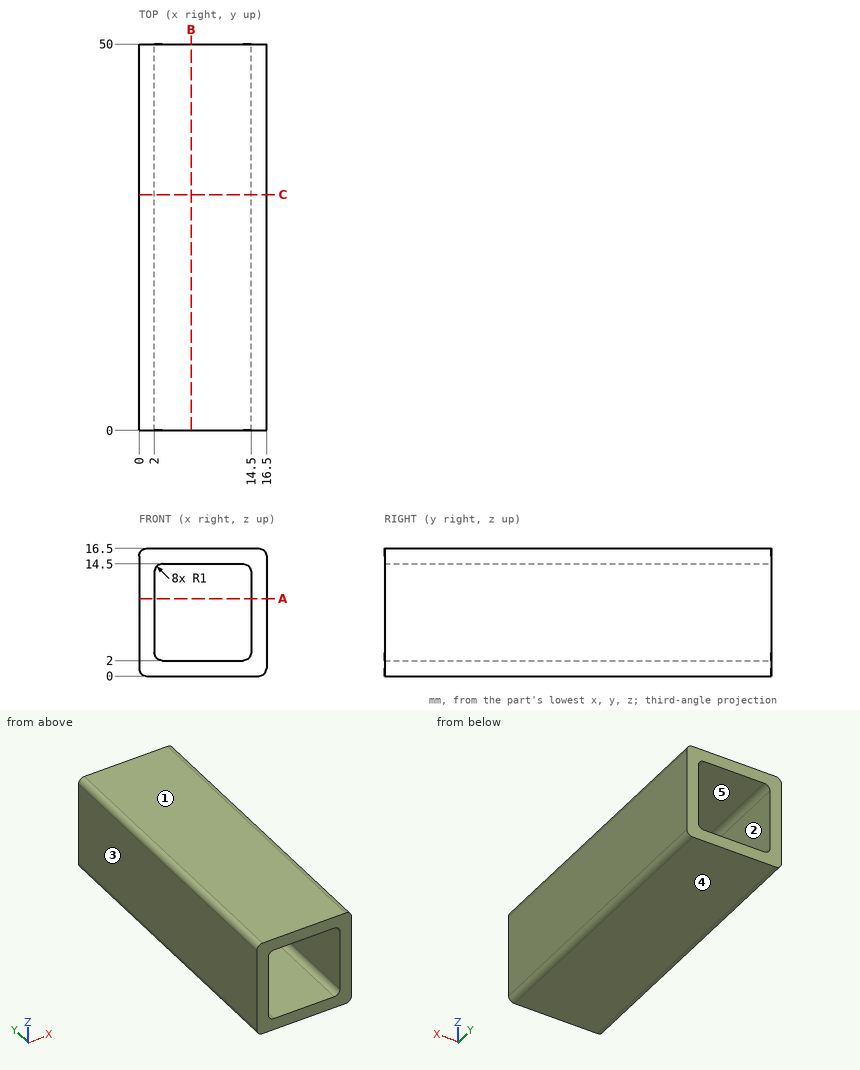
Could you check a few things on this drawing? It's one solid part, dimensions in mm from its lowest x, y, z. A direction names the side the tool comes from. Give positions to 0.01 mm unless a question says otherwise; leave off trailing zeros. Order: outer loops, then holes, each group sorted by start corner. A loop starts at its lowest first (then second) coordinate and runs counter-clockwise, first axis right, second up. Notation, with made-up numbers: M 3,21.25 L 58,21.25 A7 ccw 58,26.25 Z; hole C 74.25,71.25 d9. An arc over 180 degrees is marked long. Use one line per item in the form item = value.
Item 1: If we section it at A-A, the plane z = 10: Write out the boundary of the cut face in (x, y), and give its area (3 significant figures).
Values follow:
outline = M 0,0 L 2,0 L 2,50 L 0,50 Z; M 14.5,0 L 16.5,0 L 16.5,50 L 14.5,50 Z
area = 200 mm^2
Item 2: If we section it at C-C, the plane y = 30.5: Write out the boundary of the cut face in (x, z).
Values follow:
outline = M 0,1 A1 ccw 1,0 L 15.5,0 A1 ccw 16.5,1 L 16.5,15.5 A1 ccw 15.5,16.5 L 1,16.5 A1 ccw 0,15.5 Z; hole M 2,3 A1 ccw 3,2 L 13.5,2 A1 ccw 14.5,3 L 14.5,13.5 A1 ccw 13.5,14.5 L 3,14.5 A1 ccw 2,13.5 Z
Item 3: Will this pin go through, and if not, where does the flat tip stop? pin 1 Ø1 at (x, z) = (7, 13.5) entering from +Y.
Values follow:
pin_1 = through
Item 4: Thinking about a two-plate mould opening in Z: for the marked faces 3, 4 and 5, which applies, pulls with the +Z half, pulls with the -Z half, needs draft (parallel to the pull), parting line crosses it, or undercut?
Values follow:
face_3 = needs draft
face_4 = pulls with the -Z half
face_5 = undercut
Item 5: If we section it at B-B, the plane x = 6.75: Write out the boundary of the cut face in (y, z), and give its area (3 significant figures).
Values follow:
outline = M 0,0 L 50,0 L 50,2 L 0,2 Z; M 0,14.5 L 50,14.5 L 50,16.5 L 0,16.5 Z
area = 200 mm^2
Item 6: If I drill on line 1 along X through (y, z) = (26.5, 13.5); line 2 along Z through (x, y) = (2.25, 17), over which ranges is the centre line in solid material (lowest first)? Write a range as [from, to].
Values follow:
line_1 = [0, 2], [14.5, 16.5]
line_2 = [0, 2.34], [14.16, 16.5]
Item 7: For the marked faces 1 and 2, which set-ups out of +Z, -Z, +X, -X, +Y, -Y let a thin tool reach every point of the face, with its end or its side?
Values follow:
face_1 = +Z, +X, -X, +Y, -Y
face_2 = +Y, -Y
